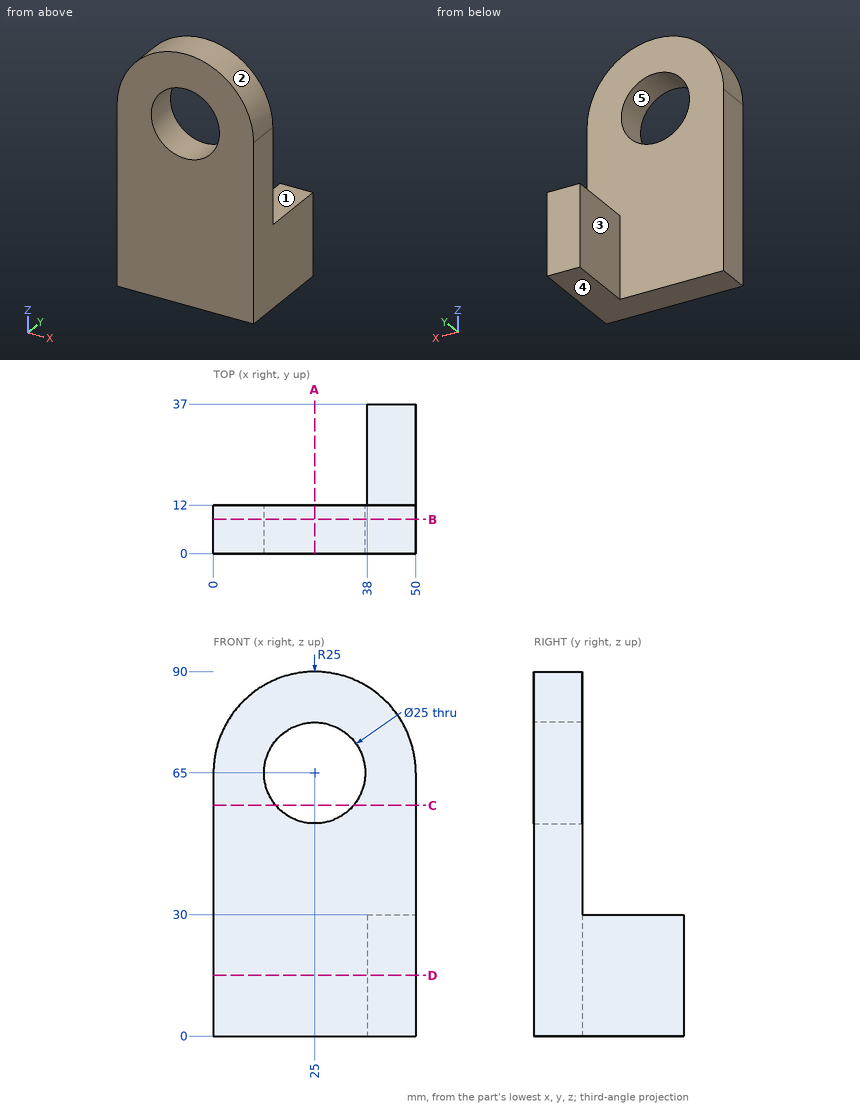
Job drawing, mm, ordinate dimensions from the low corner. One solid piece. A direction names the side the tool comes from. Give positions to 0.01 mm unless a question says otherwise; leave off trailing zeros. Write each loop counter-clockwise with the first axis right and the second up, starting at its lowest first coordinate (ties: lowest second). Pieces come first, ordered by that corner, then holes. Notation, with made-up numbers: M 44.25,30.5 L 96.25,30.5 A28 cw 96.25,64.5 Z; hole C 39,40.5 d10. An arc over 180 degrees is marked long. One line per item, written item: value. Start each with the question number.
Q1. Two-plate mould, pull along X, no slides. Class the marked faces 3, 4 and 5: +X half, -X half, draft (parallel to the pull), parting line (faces both ways), or undercut.
Q2. Saw through at D-D, the plane z = 15. Write the cut outline in (x, y).
Q3. Saw through at B-B, the plane y = 8.5. Write the cut outline in (x, z).
Q4. Probe probe 1 along X at (y, z) = (4.25, 65); probe 2 along Y at (x, z) = (41, 34); probe 3 along Z at (x, y) = (40.5, 25). List the from-to ranges inside material, lowest first. Write a range as [from, to].
Q5. Saw through at C-C, the plane z = 57. Write the cut outline in (x, y), plus the area to 3 significant figures.
Q6. Saw through at A-A, the plane x = 25. Write the cut outline in (y, z), plus the area to 3 significant figures.
Q7. Drop flat-ended pins along their axis: pin 1 Ø10 at (x, y) = (44, 15.5) entering from +Z; pin 2 Ø4 at (x, y) = (38.5, 12.5) entering from -Z; pin 3 Ø9.5 at (x, y) = (42, 24.5) entering from +Z; pin 4 Ø2 at (x, z) = (40, 53.5) entering from +Y. Give the stop position or say it passes through.
Q8. 3-axis set-ups, long thin cutter, end or side, ignore diameter. For the marked faces 1 and 2: which of +Z, -Z, +X, -X, +Y, -Y reach the whole face in a straight line?
Output values:
1. face 3: -X half
1. face 4: draft
1. face 5: undercut
2. outline: M 0,0 L 50,0 L 50,37 L 38,37 L 38,12 L 0,12 Z
3. outline: M 0,0 L 50,0 L 50,65 A25 ccw 0,65 Z; hole C 25,65 d25
4. probe 1: x = [0, 12.5], [37.5, 50]
4. probe 2: y = [0, 12]
4. probe 3: z = [0, 30]
5. outline: M 0,0 L 15.4,0 L 15.4,12 L 0,12 Z; M 34.6,0 L 50,0 L 50,12 L 34.6,12 Z
5. area: 369 mm²
6. outline: M 0,0 L 12,0 L 12,52.5 L 0,52.5 Z; M 0,77.5 L 12,77.5 L 12,90 L 0,90 Z
6. area: 780 mm²
7. pin 1: stops at z = 84.67
7. pin 2: stops at z = 0
7. pin 3: stops at z = 30
7. pin 4: stops at y = 12
8. face 1: +Z, +X, -X, +Y
8. face 2: +Z, +Y, -Y
